Study the drawing (mm; zero at the part's minimum x, y, z) and answer. Coordinates: 2 decimals unless noted, no trailing zeros. Loops run counter-clockwise (first coordinate to the right, second up) from the corner with the lowest first, then second, coordinate; pieces in that order, holes last. Notation, with made-up numbers: (-17.75, 56.25) - (-11.75, 56.25) arc R13 cw to (-11.75, 73.25) - close; hole circle Ø6 at (41.25, 80.5). An arc over 180 degrees is marked (long way). Use one line per item in the form item = value.
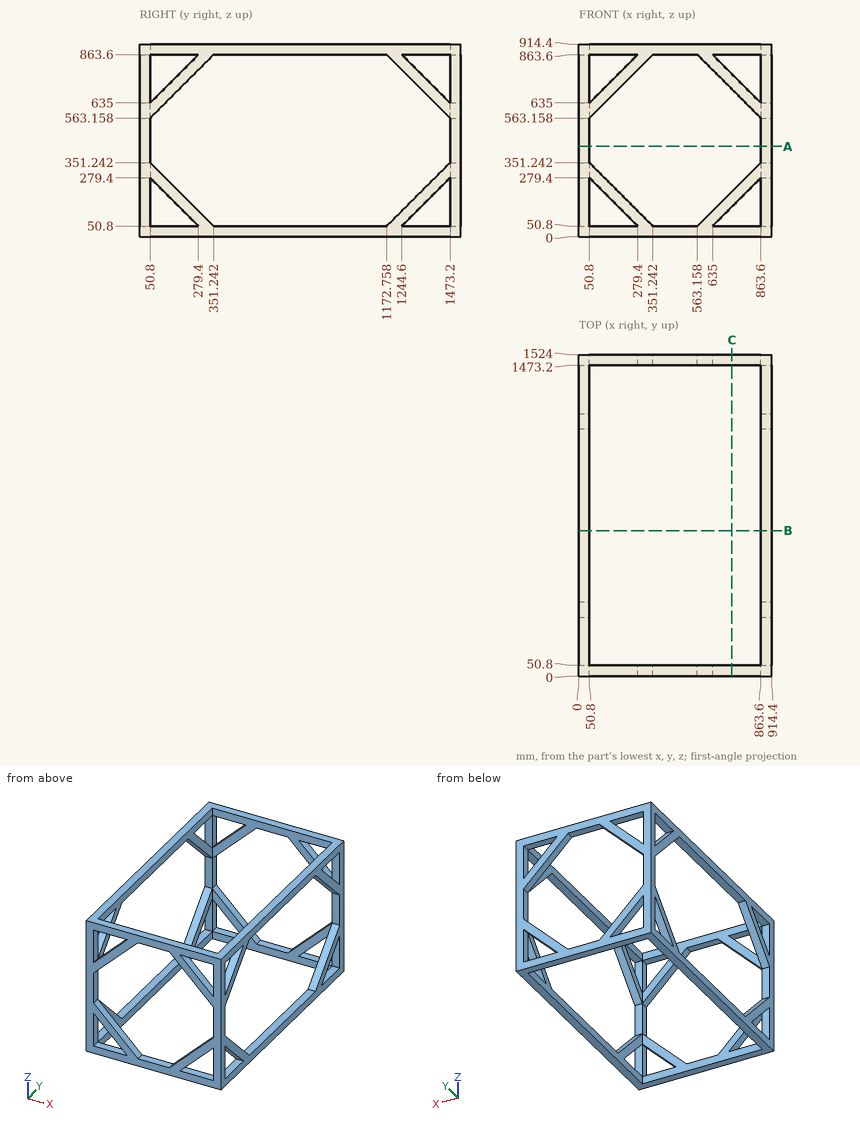
Item 1: Find the intervals of material crossed by L1, parallel to Y at x = 161.5, z = 686.5; L2, parallel to X at y = 1401, z = 40, in increasing order.
Results below:
L1 = 0 to 50.8, 1473.2 to 1524
L2 = 0 to 50.8, 863.6 to 914.4
Item 2: The part is cut by section C-C on x = 726.5. Count the separate pieces of the cut face and the enclosed holes in it, plus the area to 3 significant figures.
Results below:
separate_pieces = 8
enclosed_holes = 0
area = 24,900 mm²
Item 3: The part is cut by section B-B on y = 689.5. Give the vertices of the cut face in (x, z).
Results below:
outline = (0, 0) - (50.8, 0) - (50.8, 50.8) - (0, 50.8) - close; (0, 863.6) - (50.8, 863.6) - (50.8, 914.4) - (0, 914.4) - close; (863.6, 0) - (914.4, 0) - (914.4, 50.8) - (863.6, 50.8) - close; (863.6, 863.6) - (914.4, 863.6) - (914.4, 914.4) - (863.6, 914.4) - close
Item 4: The part is cut by section A-A on z = 428.5. Give the vertices of the cut face in (x, y), plus the area to 3 significant figures.
Results below:
outline = (0, 0) - (50.8, 0) - (50.8, 50.8) - (0, 50.8) - close; (0, 1473.2) - (50.8, 1473.2) - (50.8, 1524) - (0, 1524) - close; (863.6, 0) - (914.4, 0) - (914.4, 50.8) - (863.6, 50.8) - close; (863.6, 1473.2) - (914.4, 1473.2) - (914.4, 1524) - (863.6, 1524) - close
area = 10,300 mm²
